Can you work these out from the model? Positions are in its coordinate system, mm. A direction names the side the tool comes from. Give positions to 0.01 mm unless a question says otherwise; leave off trailing zeros. Loops run counter-clockwise (first coordinate to the right, second up) from the corner with the lowest first, then second, coordinate; pieces in that order, holes last. Notation, with made-up numbers: M 28.5,26 L 41.5,26 A24 ccw 41.5,61 Z; hole C 27.25,4 d3. An arc over 180 degrees is marked long. Answer as a JSON object with one key per item and string values.
```python
from build123d import *

# Parameters (mm, degrees)
SKETCH1_W           = 21.59
SKETCH1_H           = 46.99
BOSS_EXTRUDE1_DEPTH = 19.05
SKETCH2_R           = 2.6035
CUT_EXTRUDE1_DEPTH  = 47.99
SKETCH4_R           = 2.5527
CUT_EXTRUDE3_DEPTH  = 22.59
CUT_EXTRUDE5_DEPTH  = 5.08
SKETCH8_W           = 21.59
SKETCH8_H           = 46.99
BOSS_EXTRUDE2_DEPTH = 5.588
SKETCH9_R           = 2.0193
CUT_EXTRUDE6_DEPTH  = 5.08
CHAMFER1_SIZE       = 1.27


with BuildPart() as part:
    # Sketch1 → Boss-Extrude1 (new body, symmetric)
    with BuildSketch(Plane(origin=(0, 0, 0), x_dir=(1, 0, 0), z_dir=(0, 1, 0))):
        Rectangle(SKETCH1_W, SKETCH1_H)
    extrude(amount=BOSS_EXTRUDE1_DEPTH, both=True)

    # Sketch2 → Cut-Extrude1 (cut, through all)
    with BuildSketch(Plane.XY.offset(23.495)):
        with Locations((3.4544, -12.7)):
            Circle(SKETCH2_R)
        with Locations((3.4544, 0)):
            Circle(SKETCH2_R)
    extrude(amount=-CUT_EXTRUDE1_DEPTH, mode=Mode.SUBTRACT)

    # Sketch4 → Cut-Extrude3 (cut, through all)
    with BuildSketch(Plane(origin=(10.795, 0, 0), x_dir=(0, 0, -1), z_dir=(1, 0, 0))):
        with Locations((-12.7, 12.7)):
            Circle(SKETCH4_R)
        with Locations((12.7, 12.7)):
            Circle(SKETCH4_R)
        with Locations((0, 12.7)):
            Circle(SKETCH4_R)
    extrude(amount=-CUT_EXTRUDE3_DEPTH, mode=Mode.SUBTRACT)

    # Sketch7 → Cut-Extrude5 (cut)
    with BuildSketch(Plane(origin=(10.795, 0, 0), x_dir=(0, 0, -1), z_dir=(1, 0, 0))):
        with BuildLine():
            Line((-12.7, 17.78), (12.7, 17.78))
            ThreePointArc((12.7, 17.78), (17.78, 12.7), (12.7, 7.62))
            Line((12.7, 7.62), (-12.7, 7.62))
            ThreePointArc((-12.7, 7.62), (-17.78, 12.7), (-12.7, 17.78))
        make_face()
    extrude(amount=-CUT_EXTRUDE5_DEPTH, mode=Mode.SUBTRACT)

    # Sketch8 → Boss-Extrude2 (add)
    with BuildSketch(Plane(origin=(0, 19.05, 0), x_dir=(1, 0, 0), z_dir=(0, 1, 0))):
        Rectangle(SKETCH8_W, SKETCH8_H)
    extrude(amount=BOSS_EXTRUDE2_DEPTH)

    # Sketch9 → Cut-Extrude6 (cut)
    with BuildSketch(Plane(origin=(0, 24.638, 0), x_dir=(1, 0, 0), z_dir=(0, 1, 0))):
        with Locations((-0.2794, 12.696926228)):
            Circle(SKETCH9_R)
        with Locations((-0.2794, -12.696926228)):
            Circle(SKETCH9_R)
    extrude(amount=-CUT_EXTRUDE6_DEPTH, mode=Mode.SUBTRACT)

    # Chamfer1
    chamfer1_edges = [part.edges().sort_by_distance(p)[0] for p in [
        (10.795, 2.794, 23.495),
        (-10.795, 2.794, 23.495),
        (-10.795, 2.794, -23.495),
        (10.795, 2.794, -23.495),
    ]]
    chamfer(chamfer1_edges, length=CHAMFER1_SIZE)


solid = part.part
```
1) Suppose I cut it at D-D, the plane y = -12.7. Write out the boundary of the cut face in (x, z) (3 decimals), and give its area (3 significant figures).
Answer list:
{"outline": "M -10.795,-22.225 L -9.525,-23.495 L 0.851,-23.495 L 0.851,23.495 L -9.525,23.495 L -10.795,22.225 Z; M 6.058,-23.495 L 9.525,-23.495 L 10.795,-22.225 L 10.795,22.225 L 9.525,23.495 L 6.058,23.495 Z", "area": "767 mm^2"}
2) If we mould it in two halves opening along X, with no side actions, what happens to faces 1 (the flat face through (0, 19.558, 13)), 2 (the cylindrical face through (-2.424, 10.435, 11.522)), 3 (the flat face through (-10.15, 3.1, -22.87))? For each: +X half, -X half, draft (parallel to the pull), parting line (faces both ways), or undercut.
Answer list:
{"face 1": "undercut", "face 2": "draft", "face 3": "-X half"}
3) Suppose I cut it at B-B, the plane z = -11.5. Give the number of separate pieces and of enclosed holes in the cut face, and give its area (3 significant figures).
Answer list:
{"separate pieces": "2", "enclosed holes": "2", "area": "758 mm^2"}
4) Suppose I cut it at A-A, the plane y = 12.7. Write out the boundary of the cut face in (x, z) (3 decimals), and give its area (3 significant figures).
Answer list:
{"outline": "M -10.795,-22.225 L -9.525,-23.495 L 9.525,-23.495 L 10.795,-22.225 L 10.795,-17.78 L 5.715,-17.78 L 5.715,-15.253 L -10.795,-15.253 Z; M -10.795,-10.147 L 5.715,-10.147 L 5.715,-2.553 L -10.795,-2.553 Z; M -10.795,2.553 L 5.715,2.553 L 5.715,10.147 L -10.795,10.147 Z; M -10.795,15.253 L 5.715,15.253 L 5.715,17.78 L 10.795,17.78 L 10.795,22.225 L 9.525,23.495 L -9.525,23.495 L -10.795,22.225 Z", "area": "578 mm^2"}
5) For faces 4 (the flat face through (0, -19.05, 0)), 5 (the cylindrical face through (0.806, 22.134, -14.4)), 6 (the cylindrical face through (8.29, 12.59, 17.78)), which set-ups out of +Z, -Z, +X, -X, +Y, -Y let a thin tool reach every point of the face, with its end or its side?
Answer list:
{"face 4": "+Z, -Z, +X, -X, -Y", "face 5": "+Y", "face 6": "+X"}
6) Will these pins go through, and if not, where does the flat tip stop? pin 1 Ø5 at (y, z) = (13, -8.5) entering from +X (3 decimals); pin 2 Ø3 at (x, y) = (3.45, 0) entering from +Z.
Answer list:
{"pin 1": "x = 5.715", "pin 2": "through"}
7) Suppose I cut it at C-C, the plane x = 4.5. Write out the boundary of the cut face in (y, z) (3 decimals).
Answer list:
{"outline": "M -19.05,-23.495 L -15.084,-23.495 L -15.084,23.495 L -19.05,23.495 Z; M -10.316,-23.495 L -2.384,-23.495 L -2.384,23.495 L -10.316,23.495 Z; M 2.384,-23.495 L 24.638,-23.495 L 24.638,23.495 L 2.384,23.495 Z; hole C 12.7,-12.7 d5.105; hole C 12.7,0 d5.105; hole C 12.7,12.7 d5.105"}
8) Please list where these lines run through material, in increasing order: line 1 along Y through (x, z) = (3.25, -9); line 2 along Y through (x, z) = (7, -11.5); line 3 along Y through (x, z) = (-5.75, 0). Write a range as from..to.
Answer list:
{"line 1": "-19.05..-15.3, -10.1..-2.6, 2.6..24.64", "line 2": "-19.05..7.62, 17.78..24.64", "line 3": "-19.05..10.15, 15.25..24.64"}
